Model file for the job. Use its own axes, mm. A direction names the side the tool comes from. Coordinates: 2 decimals unless noted, no trailing zeros. Write each loop counter-clockwise with the first axis right and the second up, starting at its lowest first coordinate (ties: lowest second). Pieces come first, ordered by that corner, then holes. Notation, with made-up numbers: M -11.5,-1 L 32.5,-1 A19 cw 32.5,34 Z; hole C 43,-34 d2. An arc over 180 degrees is marked long. One line per question, with ' | ' between items. Start each with the question number.
(1) Wall check: probe 1 along Y at (x, z) = (18, 18.25); probe 2 along Z at (x, y) = (8.5, -0.25); probe 3 along Z at (x, y) = (24.5, -5.25). Give the ranges that are in metal, low to high.
(2) Tool access for faces 1 (the face through (-3, -8.329, 15)), 2 (the face through (-3, -1, 11.09)), 3 (the face through (-32.921, -5.236, 18.235)): list every direction of +Z, -Z, +X, -X, +Y, -Y with a clear straight run to the whole face (end or side of a thin tool).
(3) Flat gauge pins, fed straight in: pin 1 Ø1 at (y, z) = (-1, 15) entering from -X; pin 2 Ø1.5 at (y, z) = (-8, 17) entering from -X; pin 3 Ø0.6 at (x, y) = (6, -9.5) entering from +Z; pin 4 Ø2.5 at (x, z) = (3.5, 16.5) entering from +Y. Where does each tip first touch, or does it go through?
(4) Cut at C-C (y = -0.75). Write the cut outline in (x, z), plus the area to 4 significant figures.
(5) Cut at A-A (x = -27). Write the cut outline in (y, z).
(6) Cut at B-B (z = 12.5). Write the cut outline in (x, y).
from build123d import *

# Parameters (mm, degrees)
F1_DEPTH = 10.3
F2_W     = 2.064651
F2_H     = 8.540146
F2_W_2   = 2.228884
F2_H_2   = 8.727841
F3_DEPTH = 61.101


with BuildPart() as f1:
    # F0 (on Front) → F1 (new body)
    with BuildSketch(Plane.XZ):
        with BuildLine():
            Line((24.277063, 19.090399), (-30.822937, 19.090399))
            ThreePointArc((-30.822937, 19.090399), (-32.944257, 18.211719), (-33.822937, 16.090399))
            Line((-33.822937, 16.090399), (-33.822937, 9.590399))
            Line((-33.822937, 9.590399), (27.277063, 9.590399))
            Line((27.277063, 9.590399), (27.277063, 16.090399))
            ThreePointArc((27.277063, 16.090399), (26.398384, 18.211719), (24.277063, 19.090399))
        make_face()
    extrude(amount=F1_DEPTH)

    # F2 (on face) → F3 (cut, through all)
    with BuildSketch(Plane.YZ.offset(27.277063)):
        with Locations((-9.361314, 15.360472)):
            Rectangle(F2_W, F2_H)
        with Locations((-1.114442, 15.45432)):
            Rectangle(F2_W_2, F2_H_2)
    extrude(amount=-F3_DEPTH, mode=Mode.SUBTRACT)


solid = f1.part
Filled in:
1) probe 1: -8.33 to -2.23 | probe 2: 9.59 to 11.09 | probe 3: 9.59 to 19.08
2) face 1: +Z, +X, -X, -Y | face 2: +Z, +X, -X, +Y | face 3: +Z, -X, +Y, -Y
3) pin 1: through | pin 2: x = -33.82 | pin 3: z = 11.09 | pin 4: y = -2.23
4) outline: M -33.82,9.59 L 27.28,9.59 L 27.28,11.09 L -33.82,11.09 Z | area: 91.65 mm²
5) outline: M -10.3,9.59 L 0,9.59 L 0,11.09 L -2.23,11.09 L -2.23,19.09 L -8.33,19.09 L -8.33,11.09 L -10.3,11.09 Z
6) outline: M -33.82,-8.33 L 27.28,-8.33 L 27.28,-2.23 L -33.82,-2.23 Z
